```python
from build123d import *

# Parameters (mm, degrees)
SKETCH_1_W      = 40
SKETCH_1_H      = 30
EXTRUDE_1_DEPTH = 15
SKETCH_3_R      = 1.55
EXTRUDE_2_DEPTH = 5
SKETCH_4_W      = 6
SKETCH_4_H      = 4.77
EXTRUDE_3_DEPTH = 4


with BuildPart() as part:
    # 草图1 → 凸台-拉伸1 (new body)
    with BuildSketch(Plane.XY):
        with Locations((-64.15, 0.5)):
            Rectangle(SKETCH_1_W, SKETCH_1_H)
    extrude(amount=-EXTRUDE_1_DEPTH)

    # 草图3 → 凸台-拉伸2 (add)
    with BuildSketch(Plane(origin=(-44.15, 0, 0), x_dir=(0, 0, -1), z_dir=(1, 0, 0))):
        with BuildLine():
            Line((7.084541854, 15.5), (15, 15.5))
            Line((15, 15.5), (15, 15.003385417))
            ThreePointArc((15, 15.003385417), (18.463655357, 19.83658452), (12.644770927, 21.060229073))
            Line((12.644770927, 21.060229073), (7.084541854, 15.5))
        make_face()
        with Locations((15.155, 18.55)):
            Circle(SKETCH_3_R, mode=Mode.SUBTRACT)
    extrude_2 = extrude(amount=-EXTRUDE_2_DEPTH)

    # 镜向2: 凸台-拉伸2 across plane
    add(extrude_2.mirror(Plane.ZX.offset(0.5)))

    # 草图4 → 凸台-拉伸3 (add)
    with BuildSketch(Plane(origin=(0, 0, -15), x_dir=(-1, 0, 0), z_dir=(0, 0, -1))):
        with Locations((47.15, 13.115)):
            Rectangle(SKETCH_4_W, SKETCH_4_H)
        with Locations((81.15, 13.115)):
            Rectangle(SKETCH_4_W, SKETCH_4_H)
        with Locations((81.15, -12.115)):
            Rectangle(SKETCH_4_W, SKETCH_4_H)
        with Locations((47.15, -12.115)):
            Rectangle(SKETCH_4_W, SKETCH_4_H)
    extrude(amount=EXTRUDE_3_DEPTH)


solid = part.part
```
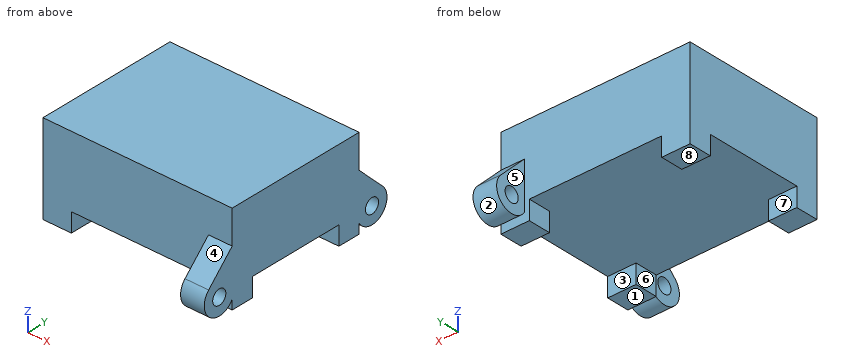
Here's how the part is built. I have some questions about the finished solid (model axes, mm). Face numbers are marked on the shaded views. A direction names the side the tool comes from. Round coordinates to 2 decimals unless told otherwise and drop trailing zeros. Write each loop counter-clockwise with the first axis right and the second up, starting at its lowest first coordinate (ties: lowest second). Pieces come first, ordered by that corner, then holes.
Q1. If we section it at D-D on z = -9: Write out the boundary of the cut face in (x, y), plus the area to 3 significant figures.
Q2. If we section it at A-A on z = -17.5: Write out the boundary of the cut face in (x, y), plus the area to 3 significant figures.
Q3. Which directions (+Z, -Z, +X, -X, +Y, -Y) give clear straight access to the entire face, cutting with the end or side of a thin tool? Please do the marked faces 5, 6, 7 and 8.
Q4. Will these pins go through, and if not, where does the flat tip stop? P1, Ø5, axis at x = -67.5, y = -16.5, coming from the -Z side; P2, Ø9.5, axis at x = -58.5, z = -11, coming from the -Y side; P3, Ø3, axis at y = -17.55, z = -15.155, coming from the -X side; P4, Ø4, axis at x = -61.5, z = -4.5, coming from the +Y side.
Q5. If we mould it in two halves opening along Y, with no side actions, what happens to the marked faces 1, 2, 3 and 4? For each: +Y half, -Y half, draft (parallel to the pull), parting line (faces both ways), or undercut.
Q6. If we section it at C-C on y = 6: Write out the boundary of the cut face in (x, z).
Q7. If we section it at B-B on y = 17.5: Write out the boundary of the cut face in (x, z), plus the area to 3 significant figures.
Q8. Please list where these lines run through material, in increasing order: probe 1 along Y at (x, z) = (-57, -5.75); probe 2 along Z at (x, y) = (-45.9, -17.55) (3 decimals); probe 3 along Z at (x, y) = (-72, -12.5).
Answer below:
1. outline: (-84.15, -14.5) - (-49.15, -14.5) - (-49.15, -16.42) - (-44.15, -16.42) - (-44.15, 17.42) - (-49.15, 17.42) - (-49.15, 15.5) - (-84.15, 15.5) - close
1. area: 1,220 mm2
2. outline: (-84.15, -14.5) - (-78.15, -14.5) - (-78.15, -9.73) - (-84.15, -9.73) - close; (-84.15, 10.73) - (-78.15, 10.73) - (-78.15, 15.5) - (-84.15, 15.5) - close; (-50.15, -14.5) - (-44.15, -14.5) - (-44.15, -9.73) - (-50.15, -9.73) - close; (-50.15, 10.73) - (-44.15, 10.73) - (-44.15, 15.5) - (-50.15, 15.5) - close; (-49.15, -20.22) - (-44.15, -20.22) - (-44.15, -14.88) - (-49.15, -14.88) - close; (-49.15, 15.88) - (-44.15, 15.88) - (-44.15, 21.22) - (-49.15, 21.22) - close
2. area: 168 mm2
3. face 5: +Z, -Z, -X, +Y
3. face 6: -Z, +Y, -Y
3. face 7: -Z, +X, -X
3. face 8: -Z, +X, -X, +Y, -Y
4. P1: stops at z = -15
4. P2: stops at y = -14.5
4. P3: passes through
4. P4: stops at y = 15.5
5. face 1: draft
5. face 2: undercut
5. face 3: undercut
5. face 4: -Y half
6. outline: (-84.15, -15) - (-44.15, -15) - (-44.15, 0) - (-84.15, 0) - close
7. outline: (-49.15, -18.55) - (-44.15, -18.55) - (-44.15, -16.3) - (-49.15, -16.3) - close; (-49.15, -14.01) - (-44.15, -14.01) - (-44.15, -9.08) - (-49.15, -9.08) - close
7. area: 35.9 mm2
8. probe 1: y = -14.5 to 15.5
8. probe 2: z = -18.705 to -16.705, -13.605 to -10.135
8. probe 3: z = -15 to 0
